Design review of the part built by this model. Coordinates are the model's own, in mm. A direction names the side the tool comes from. Round coordinates to 2 decimals unless told otherwise and drop trailing zeros. Write each loop counter-clockwise with the first axis right and the second up, starting at its lowest first coordinate (ties: lowest second). Pieces come first, ordered by that corner, then holes. Notation, with made-up numbers: (-13, 65.5) - (38, 65.5) arc R22 cw to (38, 91.5) - close; hole circle Ø3 at (5.5, 17.25). An arc over 180 degrees is marked (long way). Use one line per item in the form item = value.
```python
from build123d import *

# Parameters (mm, degrees)
HEAD_DEPTH     = 4
SHANK_SKETCH_R = 2
SHANK_DEPTH    = 25
SKETCH6_R      = 2.625
HEAD_CUT_DEPTH = 1
FILLET1_R      = 1


with BuildPart() as part:
    # Head Sketch → Head (new body)
    with BuildSketch(Plane.XY):
        Polygon((0, 4.041451884), (3.5, 2.020725942), (3.5, -2.020725942), (0, -4.041451884), (-3.5, -2.020725942), (-3.5, 2.020725942), align=None)
    extrude(amount=HEAD_DEPTH)

    # Shank Sketch → Shank (add)
    with BuildSketch(Plane.XY):
        Circle(SHANK_SKETCH_R)
    extrude(amount=-SHANK_DEPTH)

    # Sketch3 → Flange (revolve)
    with BuildSketch(Plane(origin=(0, 0, 0), x_dir=(-1, 0, 0), z_dir=(0, 1, 0)), mode=Mode.PRIVATE) as flange_sk:
        with BuildLine():
            Line((-5, 0), (0, 0))
            Line((0, 0), (0, 1.5))
            ThreePointArc((0, 1.5), (-2.562220765, 1.372207648), (-5.099009901, 0.99009901))
            ThreePointArc((-5.099009901, 0.99009901), (-5.497518595, 0.45024814), (-5, 0))
        make_face()
    revolve(flange_sk.sketch.rotate(Axis((0, 0, 0), (0, 0, 1)), 30), axis=Axis((0, 0, 0), (0, 0, 1)))

    # Sketch5 → Head Trim (revolve, cut)
    with BuildSketch(Plane(origin=(0, 0, 0), x_dir=(0, 0, -1), z_dir=(1, 0, 0)), mode=Mode.PRIVATE) as head_trim_sk:
        with BuildLine():
            Line((-4, -3.041451884), (-4, -4.041451884))
            Line((-4, -4.041451884), (-3, -4.041451884))
            ThreePointArc((-3, -4.041451884), (-3.707106781, -3.748558666), (-4, -3.041451884))
        make_face()
    revolve(head_trim_sk.sketch.rotate(Axis((0, 0, 15.085599173), (0, 0, -1)), 90), axis=Axis((0, 0, 15.085599173), (0, 0, -1)), mode=Mode.SUBTRACT)

    # Sketch6 → Head Cut (cut)
    with BuildSketch(Plane.XY.offset(4)):
        Circle(SKETCH6_R)
    extrude(amount=-HEAD_CUT_DEPTH, mode=Mode.SUBTRACT)

    # Fillet1
    fillet1_edges = [part.edges().sort_by_distance(p)[0] for p in [
        (-2.625, 0, 3),
    ]]
    fillet(fillet1_edges, radius=FILLET1_R - 0.0001)  # a hair under: the kernel refuses the full size


solid = part.part
```
Q1. To check wall thickness, follow line 1 along Z through (x, y) = (-0.25, -1.5); line 2 along X through (y, z) = (-1.5, 1.5); line 3 along Z through (x, y) = (-2.25, 4.75). State the ranges of each line that lie inside material, in increasing order. Write a range as from..to.
Calculated:
line_1 = -25..3
line_2 = -3.5..3.5
line_3 = 0.07..0.93
Q2. We need section B-B on z = -15.75. Write out the cut boundary in (x, y), then the cut area to 3 significant figures.
Calculated:
outline = circle Ø4 at (0, 0)
area = 12.6 mm2
Q3. For P1, Ø2, axis at x = -3.5, z = -12.5, coming from the -Y side; P2, Ø1, axis at y = -0.5, z = -15.5, coming from the +X side; P3, Ø2.5, axis at x = 0.5, y = -0.5, coming from the +Z side; P4, Ø3, axis at y = -0.5, z = 2, coming from the +X side, all flat-tipped, find the tip position at first contact; note any pin that passes through.
Calculated:
P1 = through
P2 = 2
P3 = 3.06
P4 = 5.5
Q4. Machinability: for faces 1 (the cylindrical face through (0, -2, -12)), 2 (the flat face through (-1.725, -3.045, 2.516)), 3 (the flat face through (1.8, -3, 2.5)), 4 (the flat face through (1.725, 3.045, 2.516)), which of the approach directions +Z, -Z, +X, -X, +Y, -Y give a long, thin tool a straight path to every point of the face, cutting with its end or side? Answer none if there is none.
Calculated:
face_1 = -Z
face_2 = +Z, -X, -Y
face_3 = +Z, +X, -Y
face_4 = +Z, +X, +Y
Q5. Draft analysis for pull direction Y (two halves, no side actions). For faces 5 (the flat face through (-1.8, 3, 2.5)), 6 (the flat face through (0, 0, 3)), 7 (the flat face through (2, 1, 0)), state which applies: released by +Y, released by -Y, zero draft, split by the parting line, or undercut.
Calculated:
face_5 = released by +Y
face_6 = undercut
face_7 = zero draft
